Geometry check sheet. Reference: drawing and pictorial views, mm from the part's lowest x, y, z. Round coordinates to 2 decimals unless told otherwise and drop trailing zeros. Order: outer loops, then holes, each group sorted by start corner. A loop starts at its lowest first (then second) coordinate and runs counter-clockwise, first axis right, second up.
(1) Thickness scan on L1, parallel to Y at x = 19.11, z = 0.8 (3 decimals); L2, parallel to Y at x = 65.5, z = 0.55; L3, parallel to X at y = 33, z = 0.3. Record the ranges inside material, lowest first.
(2) Cross-section at C-C on z = 0.4. Count the separate pieces of the cut face and the enclosed holes in it, and give its area (3 significant figures).
(3) Gauge pin test, flat end, axial feed: P1, Ø3.5, axis at x = 7.5, y = 49.75, coming from the -Z side. Record the tip position at first contact, or that the pin passes through.
(4) Cross-section at A-A on x = 19.11. Enter the section's corners in (y, z) (3 decimals), and give its area (3 significant figures).
(5) Cross-section at B-B on y = 49.75. Enter the section's corners in (x, z), and give its area (3 significant figures).
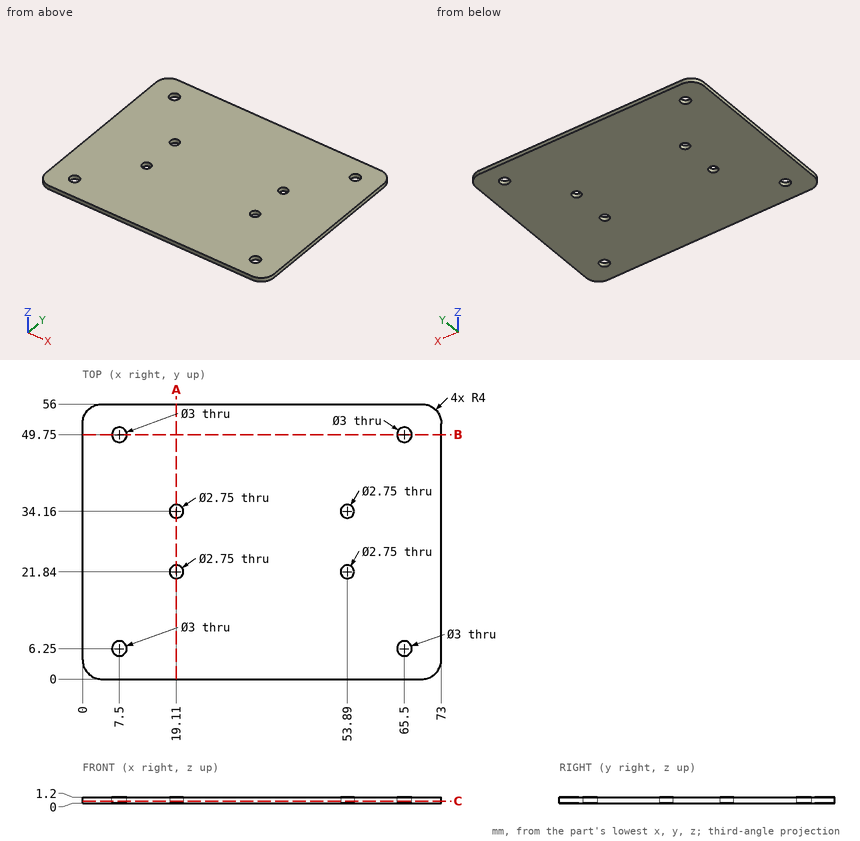
Found:
1. L1: y = 0 to 20.465, 23.215 to 32.785, 35.535 to 56
1. L2: y = 0 to 4.75, 7.75 to 48.25, 51.25 to 56
1. L3: x = 0 to 18.37, 19.85 to 53.15, 54.63 to 73
2. separate pieces: 1
2. enclosed holes: 8
2. area: 4,020 mm2
3. P1: stops at z = 0
4. outline: (0, 0) - (20.465, 0) - (20.465, 1.2) - (0, 1.2) - close; (23.215, 0) - (32.785, 0) - (32.785, 1.2) - (23.215, 1.2) - close; (35.535, 0) - (56, 0) - (56, 1.2) - (35.535, 1.2) - close
4. area: 60.6 mm2
5. outline: (0, 0) - (6, 0) - (6, 1.2) - (0, 1.2) - close; (9, 0) - (64, 0) - (64, 1.2) - (9, 1.2) - close; (67, 0) - (73, 0) - (73, 1.2) - (67, 1.2) - close
5. area: 80.4 mm2
